Geometry check sheet. Reference: the model listing, model coordinates, mm. Face numbers are marked on the shaded views. A direction names the side the tool comes from. Give positions to 0.01 mm unless a question says otherwise; leave off trailing zeros. Loops run counter-clockwise (first coordinate to the right, second up) from the corner with the lowest first, then second, coordinate; pieces in that order, holes last. Notation, with made-up numbers: (-30.5, -33.5) -> (-2.5, -33.5) arc R19 ccw to (-2.5, 2.5) -> close; hole circle Ø8 at (-39.5, 10.25). An arc over 180 degrees is marked (long way). Write item = value, one per line. Start each with the question number.
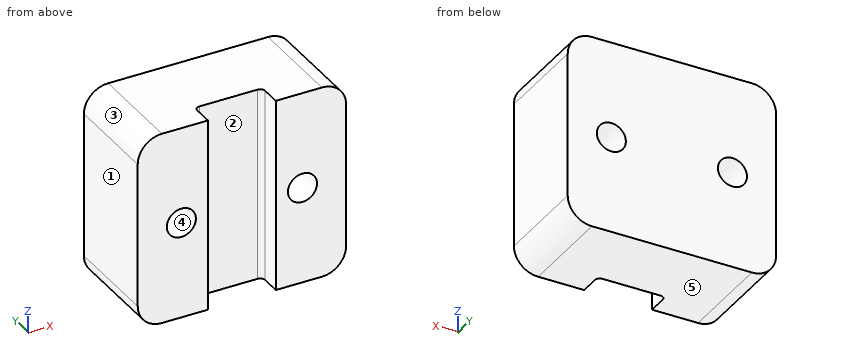
```python
from build123d import *

# Parameters (mm, degrees)
SKETCH1_W           = 43
SKETCH1_H           = 40
BOSS_EXTRUDE1_DEPTH = 20
CUT_EXTRUDE1_REACH  = 64.04
SKETCH2_R           = 3
FILLET1_R           = 5
CUT_EXTRUDE2_REACH  = 64.04
SKETCH3_W           = 14
SKETCH3_H           = 5
FILLET2_R           = 1


with BuildPart() as part:
    # Sketch1 → Boss-Extrude1 (new body)
    with BuildSketch(Plane(origin=(0, 0, 0), x_dir=(1, 0, 0), z_dir=(0, 1, 0))):
        with Locations((21.5, 20)):
            Rectangle(SKETCH1_W, SKETCH1_H)
    extrude(amount=BOSS_EXTRUDE1_DEPTH)

    # Sketch2 → Cut-Extrude1 (cut, up to next)
    with BuildSketch(Plane(origin=(0, 20, 0), x_dir=(1, 0, 0), z_dir=(0, 1, 0)), mode=Mode.PRIVATE) as cut_extrude1_sk1:
        with Locations(Location((9, 20, 0), (0, 0, 270))):
            Circle(SKETCH2_R)
    cut_extrude1_tool1 = extrude(cut_extrude1_sk1.sketch, amount=-CUT_EXTRUDE1_REACH, mode=Mode.PRIVATE) & part.part
    # Sketch2 → Cut-Extrude1 (cut, up to next)
    with BuildSketch(Plane(origin=(0, 20, 0), x_dir=(1, 0, 0), z_dir=(0, 1, 0)), mode=Mode.PRIVATE) as cut_extrude1_sk2:
        with Locations(Location((34, 20, 0), (0, 0, 270))):
            Circle(SKETCH2_R)
    cut_extrude1_tool2 = extrude(cut_extrude1_sk2.sketch, amount=-CUT_EXTRUDE1_REACH, mode=Mode.PRIVATE) & part.part
    add(cut_extrude1_tool1.solids().sort_by_distance((9, 20, -20))[0], mode=Mode.SUBTRACT)
    add(cut_extrude1_tool2.solids().sort_by_distance((34, 20, -20))[0], mode=Mode.SUBTRACT)

    # Fillet1
    fillet1_edges = [part.edges().sort_by_distance(p)[0] for p in [
        (0, 10, -40),
        (43, 10, -40),
        (43, 10, 0),
        (0, 10, 0),
    ]]
    fillet(fillet1_edges, radius=FILLET1_R)

    # Sketch3 → Cut-Extrude2 (cut, up to next)
    with BuildSketch(Plane.XY, mode=Mode.PRIVATE) as cut_extrude2_sk1:
        with Locations((21.5, 2.5)):
            Rectangle(SKETCH3_W, SKETCH3_H)
    cut_extrude2_tool1 = extrude(cut_extrude2_sk1.sketch, amount=-CUT_EXTRUDE2_REACH, mode=Mode.PRIVATE) & part.part
    add(cut_extrude2_tool1.solids().sort_by_distance((21.5, 2.5, 0))[0], mode=Mode.SUBTRACT)

    # Fillet2
    fillet2_edges = [part.edges().sort_by_distance(p)[0] for p in [
        (14.5, 5, -20),
        (28.5, 5, -20),
    ]]
    fillet(fillet2_edges, radius=FILLET2_R)


solid = part.part
```
1) Draft check along X on the marked faces 3, 4 and 5. Enter one of: released by +X, released by -X, zero draft, split by the parting line, or undercut.
2) Depth check by flat-ended pin: pin 1 Ø8 at (x, z) = (30.5, -11) entering from -Y. Enter the tip coordinate at first touch or a pass-through.
3) Section check A-A (y = 12.25). Enter the section's corners in (x, z).
4) Section check B-B (z = -20). Enter the section's corners in (x, y).
5) Tool access check on the marked faces 1 and 2. Record the directions out of +Z, -Z, +X, -X, +Y, -Y that give a thin tool (end or side, any length) a straight path to the whole face; none if there is none.
6) Thickness scan on line 1 (X direction, y = 13.25, z = -20); line 2 (Y direction, x = 22.5, z = -4); line 3 (Z direction, x = 32.5, y = 16.25). Record the ranges inside material, lowest first.
7) Section check D-D (z = -12). Enter the section's corners in (x, y), plus the area to 3 significant figures.
8) Section check C-C (x = 9). Enter the section's corners in (y, z).
Check result:
q1.face_3 = released by -X
q1.face_4 = undercut
q1.face_5 = zero draft
q2.pin_1 = 0
q3.outline = (0, -35) arc R5 ccw to (5, -40) -> (38, -40) arc R5 ccw to (43, -35) -> (43, -5) arc R5 ccw to (38, 0) -> (5, 0) arc R5 ccw to (0, -5) -> close; hole circle Ø6 at (9, -20); hole circle Ø6 at (34, -20)
q4.outline = (0, 0) -> (6, 0) -> (6, 20) -> (0, 20) -> close; (12, 0) -> (14.5, 0) -> (14.5, 4) arc R1 cw to (15.5, 5) -> (27.5, 5) arc R1 cw to (28.5, 4) -> (28.5, 0) -> (31, 0) -> (31, 20) -> (12, 20) -> close; (37, 0) -> (43, 0) -> (43, 20) -> (37, 20) -> close
q5.face_1 = +Z, -Z, -X, +Y, -Y
q5.face_2 = +Z, -Z, -Y
q6.line_1 = 0 to 6, 12 to 31, 37 to 43
q6.line_2 = 5 to 20
q6.line_3 = -40 to -22.6, -17.4 to 0
q7.outline = (0, 0) -> (14.5, 0) -> (14.5, 4) arc R1 cw to (15.5, 5) -> (27.5, 5) arc R1 cw to (28.5, 4) -> (28.5, 0) -> (43, 0) -> (43, 20) -> (0, 20) -> close
q7.area = 790 mm2
q8.outline = (0, -40) -> (20, -40) -> (20, -23) -> (0, -23) -> close; (0, -17) -> (20, -17) -> (20, 0) -> (0, 0) -> close
